Geometry check sheet. Reference: the model listing, model coordinates, mm. A direction names the side the tool comes from. Coordinates: 2 decimals unless noted, no trailing zeros. Loops run counter-clockwise (first coordinate to the right, second up) from the corner with the lowest first, then second, coordinate; pieces in that order, holes last. Notation, with made-up numbers: (-23.5, 30) -> (2.5, 30) arc R6 ccw to (2.5, 34) -> close; hole circle Ø5 at (26, -38.75). An arc over 180 degrees is marked (long way). Answer as a JSON object with one key per item and string values.
from build123d import *

# Parameters (mm, degrees)
ESQUISSE1_W              = 40
ESQUISSE1_H              = 40
BOSS_EXTRU_1_DEPTH       = 50
ESQUISSE2_R              = 5
ENL_V_MAT_EXTRU_1_DEPTH  = 41
ESQUISSE3_R              = 5
ENL_V_MAT_EXTRU_2_DEPTH  = 41
ESQUISSE4_W              = 20
ESQUISSE4_H              = 14
ENL_V_MAT_EXTRU_3_DEPTH  = 29
ESQUISSE5_W              = 14
ESQUISSE5_H              = 20
ENL_V_MAT_EXTRU_4_DEPTH  = 29
ESQUISSE6_W              = 22
ESQUISSE6_H              = 14
ENL_V_MAT_EXTRU_5_DEPTH  = 24
ESQUISSE7_W              = 14
ESQUISSE7_H              = 22
ENL_V_MAT_EXTRU_6_DEPTH  = 24
ESQUISSE8_R              = 11
ENL_V_MAT_EXTRU_7_DEPTH  = 7
ESQUISSE9_R              = 12.5
ENL_V_MAT_EXTRU_8_DEPTH  = 1.5
ESQUISSE10_R             = 11
ENL_V_MAT_EXTRU_9_DEPTH  = 7
ESQUISSE11_R             = 12.5
ENL_V_MAT_EXTRU_10_DEPTH = 1.5
BOSS_EXTRU_2_DEPTH       = 20


with BuildPart() as part:
    # Esquisse1 → Boss.-Extru.1 (new body)
    with BuildSketch(Plane.XY):
        with Locations((-20, 20)):
            Rectangle(ESQUISSE1_W, ESQUISSE1_H)
    extrude(amount=BOSS_EXTRU_1_DEPTH)

    # Esquisse2 → Enlèv. mat.-Extru.1 (cut, through all)
    with BuildSketch(Plane(origin=(0, 40, 0), x_dir=(1, 0, 0), z_dir=(0, 1, 0))):
        with Locations(Location((-20, -15, 0), (0, 0, 270))):  # turned: the seam where the file's is
            Circle(ESQUISSE2_R)
    extrude(amount=-ENL_V_MAT_EXTRU_1_DEPTH, mode=Mode.SUBTRACT)

    # Esquisse3 → Enlèv. mat.-Extru.2 (cut, through all)
    with BuildSketch(Plane.ZY.offset(40)):
        with Locations((35, 20)):
            Circle(ESQUISSE3_R)
    extrude(amount=-ENL_V_MAT_EXTRU_2_DEPTH, mode=Mode.SUBTRACT)

    # Esquisse4 → Enlèv. mat.-Extru.3 (cut)
    with BuildSketch(Plane.ZY.offset(40)):
        with Locations((15, 20)):
            Rectangle(ESQUISSE4_W, ESQUISSE4_H)
    extrude(amount=-ENL_V_MAT_EXTRU_3_DEPTH, mode=Mode.SUBTRACT)

    # Esquisse5 → Enlèv. mat.-Extru.4 (cut)
    with BuildSketch(Plane.XZ):
        with Locations((-20, 35)):
            Rectangle(ESQUISSE5_W, ESQUISSE5_H)
    extrude(amount=-ENL_V_MAT_EXTRU_4_DEPTH, mode=Mode.SUBTRACT)

    # Esquisse6 → Enlèv. mat.-Extru.5 (cut)
    with BuildSketch(Plane(origin=(0, 0, 0), x_dir=(0, 0, -1), z_dir=(1, 0, 0))):
        with Locations((-11, 20)):
            Rectangle(ESQUISSE6_W, ESQUISSE6_H)
    extrude(amount=-ENL_V_MAT_EXTRU_5_DEPTH, mode=Mode.SUBTRACT)

    # Esquisse7 → Enlèv. mat.-Extru.6 (cut)
    with BuildSketch(Plane(origin=(0, 40, 0), x_dir=(1, 0, 0), z_dir=(0, 1, 0))):
        with Locations((-20, -39)):
            Rectangle(ESQUISSE7_W, ESQUISSE7_H)
    extrude(amount=-ENL_V_MAT_EXTRU_6_DEPTH, mode=Mode.SUBTRACT)

    # Esquisse8 → Enlèv. mat.-Extru.7 (cut)
    with BuildSketch(Plane(origin=(0, 0, 0), x_dir=(0, 0, -1), z_dir=(1, 0, 0))):
        with Locations(Location((-35, 20, 0), (0, 0, 90))):  # turned: the seam where the file's is
            Circle(ESQUISSE8_R)
    extrude(amount=-ENL_V_MAT_EXTRU_7_DEPTH, mode=Mode.SUBTRACT)

    # Esquisse9 → Enlèv. mat.-Extru.8 (cut)
    with BuildSketch(Plane(origin=(0, 0, 0), x_dir=(0, 0, -1), z_dir=(1, 0, 0))):
        with Locations(Location((-35, 20, 0), (0, 0, 90))):  # turned: the seam where the file's is
            Circle(ESQUISSE9_R)
    extrude(amount=-ENL_V_MAT_EXTRU_8_DEPTH, mode=Mode.SUBTRACT)

    # Esquisse10 → Enlèv. mat.-Extru.9 (cut)
    with BuildSketch(Plane(origin=(0, 40, 0), x_dir=(1, 0, 0), z_dir=(0, 1, 0))):
        with Locations(Location((-20, -15, 0), (0, 0, 270))):  # turned: the seam where the file's is
            Circle(ESQUISSE10_R)
    extrude(amount=-ENL_V_MAT_EXTRU_9_DEPTH, mode=Mode.SUBTRACT)

    # Esquisse11 → Enlèv. mat.-Extru.10 (cut)
    with BuildSketch(Plane(origin=(0, 40, 0), x_dir=(1, 0, 0), z_dir=(0, 1, 0))):
        with Locations(Location((-20, -15, 0), (0, 0, 270))):  # turned: the seam where the file's is
            Circle(ESQUISSE11_R)
    extrude(amount=-ENL_V_MAT_EXTRU_10_DEPTH, mode=Mode.SUBTRACT)

    # Esquisse13 → Boss.-Extru.2 (add)
    with BuildSketch(Plane.XY.offset(50)):
        Polygon((-40, 10), (-30, 10), (-30, 0), (-28, 0), (-28, 12), (-40, 12), align=None)
    extrude(amount=BOSS_EXTRU_2_DEPTH)


solid = part.part
1. Section check C-C, the plane x = -20. State how many separate pieces and enclosed holes the cut face has, then the cut area to 4 significant figures.
Evaluation:
{"separate pieces": "5", "enclosed holes": "0", "area": "414.5 mm^2"}
2. Depth check by flat-ended pin: P1, Ø5, axis at x = -35.5, y = 6.5, coming from the +Z side; P2, Ø2.5, axis at x = -22, z = 48.5, coming from the +Y side; P3, Ø3, axis at y = 3, z = 61, coming from the -X side. Enter the tip coordinate at first touch or a pass-through.
Evaluation:
{"P1": "stops at z = 50", "P2": "stops at y = 16", "P3": "stops at x = -30"}
3. Thickness scan on probe 1 along X at (y, z) = (39.3, 15); probe 2 along X at (y, z) = (27.5, 37.5); probe 3 along Y at (x, z) = (-29.5, 14.5). Record the ranges inside material, lowest first. Write a range as from..to.
Evaluation:
{"probe 1": "x = -40..-32.5, -7.5..0", "probe 2": "x = -40..-27, -13..-7", "probe 3": "y = 0..13, 27..33"}
4. Tool access check on faces 1 (the face through (-30, 5, 60)), 2 (the face through (-20, 8, 45)), 3 (the face through (-20, 35, 28)). Record the directions out of +Z, -Z, +X, -X, +Y, -Y that give a thin tool (end or side, any length) a straight path to the whole face; none if there is none.
Evaluation:
{"face 1": "+Z, -X, -Y", "face 2": "+Y, -Y", "face 3": "+Z, +Y, -Y"}
5. Mould release check, pull along X, two halves, no side actions. Record for faces 4 (the face through (-28, 6, 60)), 5 (the face through (-20, 6, 25)), 6 (the face through (-20, 28, 25)), 7 (the face through (-34, 20, 25)): released by +X, released by -X, zero draft, split by the parting line, or undercut.
Evaluation:
{"face 4": "released by +X", "face 5": "undercut", "face 6": "undercut", "face 7": "zero draft"}
6. Section check B-B, the plane y = 37. Record the boundary of the cut face in (x, z), then the cut area to 3 significant figures.
Evaluation:
{"outline": "(-40, 0) -> (0, 0) -> (0, 50) -> (-13, 50) -> (-13, 28) -> (-27, 28) -> (-27, 50) -> (-40, 50) -> close; hole circle Ø22 at (-20, 15)", "area": "1,310 mm^2"}
7. Section check A-A, the plane z = 35. Record the boundary of the cut face in (x, y), then the cut area to 4 significant figures.
Evaluation:
{"outline": "(-40, 0) -> (-27, 0) -> (-27, 15) -> (-40, 15) -> close; (-40, 25) -> (-27, 25) -> (-27, 40) -> (-40, 40) -> close; (-13, 0) -> (0, 0) -> (0, 7.5) -> (-1.5, 7.5) -> (-1.5, 9) -> (-7, 9) -> (-7, 15) -> (-13, 15) -> close; (-13, 25) -> (-7, 25) -> (-7, 31) -> (-1.5, 31) -> (-1.5, 32.5) -> (0, 32.5) -> (0, 40) -> (-13, 40) -> close", "area": "691.5 mm^2"}
